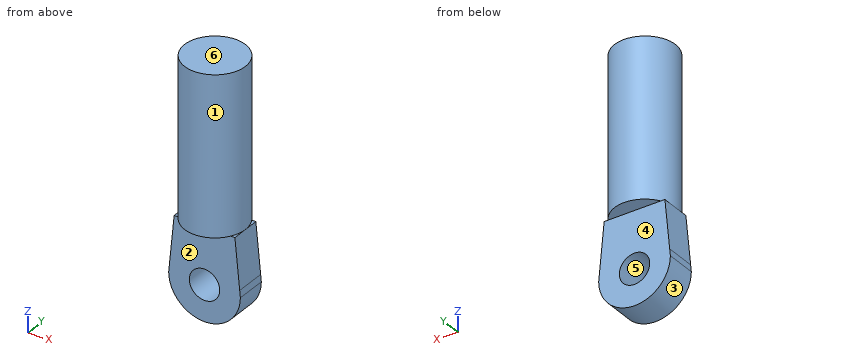
```python
from build123d import *

# Parameters (mm, degrees)
SKETCH_1_R           = 10
EXTRUDE_1_DEPTH      = 52
SKETCH_2_R           = 5
EXTRUDE_2_DEPTH      = 5
EXTRUDE_2_DEPTH_BACK = 5


with BuildPart() as part:
    # Sketch 1 → Extrude 1 (new body)
    with BuildSketch(Plane.XY):
        Circle(SKETCH_1_R)
    extrude(amount=EXTRUDE_1_DEPTH)

    # Sketch 2 → Extrude 2 (add, two sides)
    with BuildSketch(Plane(origin=(0, 0, 0), x_dir=(1, 0, 0), z_dir=(0, 1, 0))) as extrude_2_sk:
        with BuildLine():
            ThreePointArc((11.798274507, 18.566546971), (0, 30.364821478), (-11.798274507, 18.566546971))
            Line((-11.798274507, 18.566546971), (-11.578972273, 16.302329128))
            Line((-11.578972273, 16.302329128), (-10, 0))
            Line((-10, 0), (10, 0))
            Line((10, 0), (11.578972273, 16.302329128))
            Line((11.578972273, 16.302329128), (11.798274507, 18.566546971))
        make_face()
        with Locations((0, 18.566546971)):
            Circle(SKETCH_2_R, mode=Mode.SUBTRACT)
    extrude(amount=EXTRUDE_2_DEPTH)
    extrude(extrude_2_sk.sketch, amount=-EXTRUDE_2_DEPTH_BACK)


solid = part.part
```
The model under review builds one solid part; all positions refer to its coordinate system, in mm. Face numbers are marked on the shaded views. A direction names the side the tool comes from. Give positions to 0.01 mm unless a question says otherwise; leave off trailing zeros. Write each loop counter-clockwise with the first axis right and the second up, starting at its lowest first coordinate (ties: lowest second). Pieces come first, ordered by that corner, then holes.
(1) Consider section A-A, the plane x = 0. Give the boundary of the cut face in (y, z), and give its area (3 significant figures).
(2) For P1, Ø11.5, axis at x = 0, z = -18.57, coming from the +Y side; P2, Ø2.5, axis at x = 0, y = -6.5, coming from the -Z side; P3, Ø3, axis at x = 1, z = -5.5, coming from the -Y side, all flat-tipped, find the tip position at first contact; note any pin that passes through.
(3) Tool access review of the marked faces 1 and 2: name each direction out of +Z, -Z, +X, -X, +Y, -Y from which nothing blocks a thin tool from reaching the whole face with its end or side.
(4) Consider section C-C, the plane z = 5. Give the boundary of the cut face in (x, y), and give its area (3 significant figures).
(5) The part is to be moulded in two halves that separate along Z. For the marked faces 3, 4, 5 and 6, say which applies: released by +Z, released by -Z, zero draft, split by the parting line, or undercut.
(6) Consider section D-D, the plane x = -7.75. Give the boundary of the cut face in (y, z).
(7) To check wall thickness, follow L1, parallel to Y at x = -2.5, z = -9; L2, parallel to Z at x = 0, y = 0.75; L3, parallel to Z at x = -2, y = -6.25. State the ranges of each line that lie inside material, in increasing order.
Returned:
1. outline: (-10, 0) - (-5, 0) - (-5, -13.57) - (5, -13.57) - (5, 0) - (10, 0) - (10, 52) - (-10, 52) - close; (-5, -30.36) - (5, -30.36) - (5, -23.57) - (-5, -23.57) - close
1. area: 1,240 mm2
2. P1: stops at y = 5
2. P2: stops at z = 0
2. P3: stops at y = -5
3. face 1: +Z
3. face 2: -Z, +X, -X, -Y
4. outline: circle Ø20 at (0, 0)
4. area: 314 mm2
5. face 3: released by -Z
5. face 4: zero draft
5. face 5: undercut
5. face 6: released by +Z
6. outline: (-6.32, 0) - (-5, 0) - (-5, -27.46) - (5, -27.46) - (5, 0) - (6.32, 0) - (6.32, 52) - (-6.32, 52) - close
7. L1: y = -5 to 5
7. L2: z = -30.36 to -23.57, -13.57 to 52
7. L3: z = 0 to 52
